Input: part model. Units: mm. Frame: model coordinates. A direction names the side the tool comes from. Coordinates: 2 decimals unless noted, no trailing zeros. Write each loop counter-clockwise with the first axis right and the second up, starting at its lowest first coordinate (ties: lowest second). Pieces come first, ordered by that corner, then holes.
from build123d import *

# Parameters (mm, degrees)
CUT_EXTRUDE1_DEPTH      = 241
CUT_EXTRUDE1_DEPTH_BACK = 241
SKETCH4_R               = 62.5
CUT_EXTRUDE2_DEPTH      = 241.0000001
CUT_EXTRUDE2_DEPTH_BACK = 241.0000001
BOSS_EXTRUDE1_REACH     = 122
SKETCH5_R               = 72.5
SKETCH5_R_2             = 62.5


with BuildPart() as part:
    # Sketch1 → Revolve2 (revolve)
    with BuildSketch(Plane.XY):
        with BuildLine():
            Line((0, 625), (0, 605))
            ThreePointArc((0, 605), (115.458447667, 587.035007786), (220, 534.838667697))
            Line((220, 534.838667697), (220, 515))
            Line((220, 515), (195, 515))
            Line((195, 515), (195, 455))
            Line((195, 455), (195, 395))
            Line((195, 395), (220, 395))
            Line((220, 395), (220, 0))
            Line((220, 0), (240, 0))
            Line((240, 0), (240, 415))
            Line((240, 415), (215, 415))
            Line((215, 415), (215, 440))
            Line((215, 440), (240, 440))
            Line((240, 440), (240, 470))
            Line((240, 470), (215, 470))
            Line((215, 470), (215, 495))
            Line((215, 495), (240, 495))
            Line((240, 495), (240, 545))
            ThreePointArc((240, 545), (126.491106407, 604.47331922), (0, 625))
        make_face()
    revolve(axis=Axis((0, 625, 0), (0, -1, 0)))

    # Sketch2 → Cut-Extrude1 (cut, two sides)
    with BuildSketch(Plane.XY) as cut_extrude1_sk:
        with BuildLine():
            Line((-190, 0), (190, 0))
            ThreePointArc((190, 0), (0, 99.55454139), (-190, 0))
        make_face()
    extrude(amount=CUT_EXTRUDE1_DEPTH, mode=Mode.SUBTRACT)
    extrude(cut_extrude1_sk.sketch, amount=-CUT_EXTRUDE1_DEPTH_BACK, mode=Mode.SUBTRACT)

    # Sketch4 → Cut-Extrude2 (cut, two sides)
    with BuildSketch(Plane.XY) as cut_extrude2_sk:
        with Locations((0, 305)):
            Circle(SKETCH4_R)
    extrude(amount=CUT_EXTRUDE2_DEPTH, mode=Mode.SUBTRACT)
    extrude(cut_extrude2_sk.sketch, amount=-CUT_EXTRUDE2_DEPTH_BACK, mode=Mode.SUBTRACT)

    # Sketch5 → Boss-Extrude1 (add, up to next)
    with BuildSketch(Plane.XY.offset(120), mode=Mode.PRIVATE) as boss_extrude1_sk1:
        with Locations((0, 305)):
            Circle(SKETCH5_R)
        with Locations((0, 305)):
            Circle(SKETCH5_R_2, mode=Mode.SUBTRACT)
    boss_extrude1_tool1 = extrude(boss_extrude1_sk1.sketch, amount=BOSS_EXTRUDE1_REACH, mode=Mode.PRIVATE) - part.part
    add(boss_extrude1_tool1.solids().sort_by_distance((-70.44939, 305, 120))[0])

    # Mirror1: part across plane


with BuildPart() as part_1:
    add(part.part)
    add(part.part.mirror(Plane.XY))


solid = part_1.part
Item 1: Section query B-B, the plane y = 305. Return loops of the section in (x, z).
Item 2: Pin query (flat end, axial travel): pin 1 Ø6 at (x, y) = (-15, 167.5) entering from -Z; pin 2 Ø2 at (x, y) = (-185, 395.5) entering from -Z; pin 3 Ø1 at (x, z) = (74, -84.5) entering from -Y. Return the tip coordinate at first contact, or that it passes through.
Item 3: Access query for faces 4 (the face through (21.1, 364.4, -120)), 5 (the face through (-47.69, 524.78, -214.77)), 6 (the face through (17.547, 98.887, 222.967)). Directions: +Z, -Z, +X, -X, +Y, -Y. A direction counts if a zero-diameter tool reaches every point of the face in a straight line with its end or side. Return the directions, or none.
Item 4: Material intervals for line 1 (Z direction, x = 0, y = 170); line 2 (Y direction, x = 0, z = -177.5); line 3 (X direction, y = 305, z = -163), sorted ascending.
Item 5: Pull-direction query (X, two-part tool) for faces 1 (the face through (110.75, 210.4, -212.92)), 2 (the face through (221, 0, 2)), 3 (the face through (21.1, 364.4, 120)); classes: released by +X, released by -X, zero draft, split by the parting line, or undercut.
Item 6: Section query A-A, the plane z = -173. State how many separate pieces and enclosed holes the cut face has, then the cut area to 3 significant figures.
The answers:
1. outline: (-72.5, -207.71) arc R220 cw to (-72.5, 207.71) - (-72.5, 120) - (-62.5, 120) - (-62.5, 231.72) arc R240 ccw to (-62.5, -231.72) - (-62.5, -120) - (-72.5, -120) - close; (62.5, -231.72) arc R240 ccw to (62.5, 231.72) - (62.5, 120) - (72.5, 120) - (72.5, 207.71) arc R220 cw to (72.5, -207.71) - (72.5, -120) - (62.5, -120) - close
2. pin 1: stops at z = -239.7
2. pin 2: stops at z = -154.09
2. pin 3: stops at y = 587.87
3. face 4: -Y
3. face 5: none
3. face 6: +Z, -Z, -Y
4. line 1: z = -240 to -220, 220 to 240
4. line 2: y = 232.5 to 242.5, 367.5 to 377.5, 561 to 583.46
4. line 3: x = -176.16 to -147.75, -72.5 to -62.5, 62.5 to 72.5, 147.75 to 176.16
5. face 1: split by the parting line
5. face 2: zero draft
5. face 3: undercut
6. separate pieces: 2
6. enclosed holes: 1
6. area: 48,600 mm2
